The model under review builds one solid part; all positions refer to its coordinate system, in mm. Face numbers are marked on the shaded views. A direction names the side the tool comes from. Coordinates: 2 decimals unless noted, no trailing zeros. Write each loop counter-clockwise with the first axis right and the second up, starting at its lowest first coordinate (ties: lowest second). Pieces come first, ordered by that corner, then holes. Notation, with made-up numbers: (41, -34.75) -> (70, -34.75) arc R16 ccw to (70, -27.75) -> close; hole circle Ø1 at (85, 21.25). An arc over 180 degrees is marked (long way). Write each question's results on one line, items separated by ' | '.
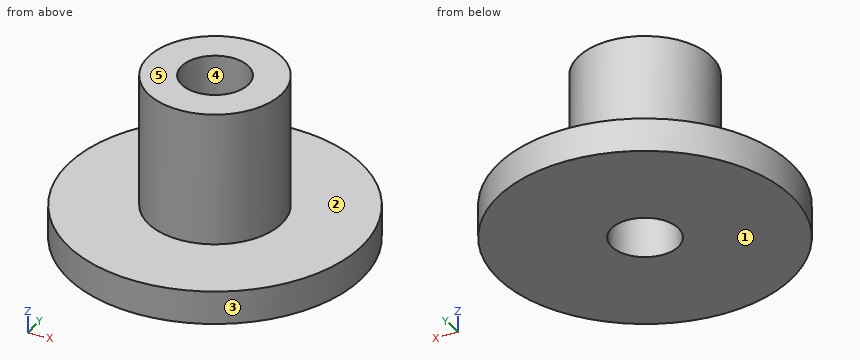
Autodesk Inventor part; units mm, degrees
ref_plane "YZ Plane" through (0, 0, 0) normal (1, 0, 0) x (0, 1, 0)
ref_plane "XZ Plane" through (0, 0, 0) normal (0, 1, 0) x (-1, 0, 0)
ref_plane "XY Plane" through (0, 0, 0) normal (0, 0, 1) x (1, 0, 0)
sketch "Эскиз1" plane through (0, 0, 0) normal (0, 0, 1) x (1, 0, 0)
  circle A0 centre (0, 0) radius 5
  dimension "d1" = 10
extrude "Выдавливание1" add sketch "Эскиз1" along normal blind 10
sketch "Эскиз2" plane through (0, 0, 0) normal (0, 0, -1) x (-1, 0, 0)
  circle A0 centre (0, 0) radius 11
  dimension "d4" = 22
extrude "Выдавливание2" add sketch "Эскиз2" along normal blind 2.5
sketch "Эскиз3" plane through (0, 0, 10) normal (0, 0, 1) x (1, 0, 0)
  circle A0 centre (0, 0) radius 2.5
  dimension "d7" = 5
extrude "Выдавливание3" cut sketch "Эскиз3" against normal blind 12.5
sketch "Эскиз4" plane through (0, 0, 0) normal (0, 0, 1) x (1, 0, 0)
  point P0 (0, 0)
properties part number "akfytw2"
Q1. Draft analysis for pull direction Y (two halves, no side actions). For the marked faces 3, 4 and 5, state which applies: pulls with the +Y half, pulls with the -Y half, needs draft (parallel to the pull), parting line crosses it, or undercut.
Solution:
face 3: parting line crosses it | face 4: undercut | face 5: needs draft
Q2. Add section D-D (x = 3.75). Write out the cut boundary in (y, z), plus the area to 3 significant figures.
Solution:
outline: (-10.34, -2.5) -> (10.34, -2.5) -> (10.34, 0) -> (3.31, 0) -> (3.31, 10) -> (-3.31, 10) -> (-3.31, 0) -> (-10.34, 0) -> close | area: 118 mm²
Q3. Add section A-A (x = 0). Write out the cut boundary in (y, z), plus the area to 3 significant figures.
Solution:
outline: (-11, -2.5) -> (-2.5, -2.5) -> (-2.5, 10) -> (-5, 10) -> (-5, 0) -> (-11, 0) -> close; (2.5, -2.5) -> (11, -2.5) -> (11, 0) -> (5, 0) -> (5, 10) -> (2.5, 10) -> close | area: 92.5 mm²
Q4. Add section C-C (z = 6.75). Write out the cut boundary in (x, y).
Solution:
outline: circle Ø10 at (0, 0); hole circle Ø5 at (0, 0)
Q5. Clearance check with flat-ended pins moving along their axes: P1, Ø5, axis at x = 0.5, z = 3, coming from the -Y side; P2, Ø6, axis at y = -5, z = 7, coming from the -X side; P3, Ø10, axis at x = -7.5, y = -8.5, coming from the +Z side. State where each tip first meets the part, or that it passes through.
Solution:
P1: y = -5 | P2: x = -4.58 | P3: z = 0
Q6. Machinability: for the marked faces 1 and 2, which of the approach directions +Z, -Z, +X, -X, +Y, -Y give a long, thin tool a straight path to every point of the face, cutting with its end or side? Answer none if there is none.
Solution:
face 1: -Z, +X, -X, +Y, -Y | face 2: +Z
Q7. For line 1 (Y direction, x = 0, z = 4.25); line 2 (Z direction, x = -6, y = 0.75); line 3 (X direction, y = -0.5, z = 0.5), list the stretches that pass through material, from the lowest coordinate up. Write a range as from..to.
Solution:
line 1: -5..-2.5, 2.5..5 | line 2: -2.5..0 | line 3: -4.97..-2.45, 2.45..4.97
